```python
from build123d import *

# Parameters (mm, degrees)
SKETCH2_W           = 75
SKETCH2_H           = 50
BOSS_EXTRUDE1_DEPTH = 101.6
CUT_EXTRUDE1_DEPTH  = 101.6
CUT_EXTRUDE2_DEPTH  = 101.6
SKETCH5_W           = 20
SKETCH5_H           = 40
CUT_EXTRUDE3_DEPTH  = 10
SKETCH6_W           = 20
SKETCH6_H           = 40
CUT_EXTRUDE4_DEPTH  = 10
SKETCH7_R           = 2.5
CUT_EXTRUDE5_DEPTH  = 2.5
SKETCH8_R           = 2.5
CUT_EXTRUDE6_DEPTH  = 2.5
CUT_EXTRUDE7_DEPTH  = 121.365392665


with BuildPart() as part:
    # Sketch2 → Boss-Extrude1 (new body)
    with BuildSketch(Plane.XY):
        with Locations((-3.307692308, -6.81353022)):
            Rectangle(SKETCH2_W, SKETCH2_H)
    extrude(amount=BOSS_EXTRUDE1_DEPTH)

    # Sketch3 → Cut-Extrude1 (cut)
    with BuildSketch(Plane(origin=(0, 18.18646978, 0), x_dir=(1, 0, 0), z_dir=(0, 1, 0))):
        Polygon((-40.807692308, -7.5), (-20.807692308, -7.5), (-7.507692308, -20.8), (-7.507692308, -80.8), (-20.807692308, -94.1), (-40.807692308, -94.1), align=None)
    extrude(amount=-CUT_EXTRUDE1_DEPTH, mode=Mode.SUBTRACT)

    # Sketch4 → Cut-Extrude2 (cut)
    with BuildSketch(Plane(origin=(0, 18.18646978, 0), x_dir=(1, 0, 0), z_dir=(0, 1, 0))):
        Polygon((34.192307692, -94.1), (14.192307692, -94.1), (0.892307692, -80.8), (0.892307692, -20.8), (14.192307692, -7.5), (34.192307692, -7.5), align=None)
    extrude(amount=-CUT_EXTRUDE2_DEPTH, mode=Mode.SUBTRACT)

    # Sketch5 → Cut-Extrude3 (cut)
    with BuildSketch(Plane.XY.offset(101.6)):
        with Locations((24.192307692, -6.81353022)):
            Rectangle(SKETCH5_W, SKETCH5_H)
    extrude(amount=-CUT_EXTRUDE3_DEPTH, mode=Mode.SUBTRACT)

    # Sketch6 → Cut-Extrude4 (cut)
    with BuildSketch(Plane.XY.offset(101.6)):
        with Locations((-30.807692308, -6.81353022)):
            Rectangle(SKETCH6_W, SKETCH6_H)
    extrude(amount=-CUT_EXTRUDE4_DEPTH, mode=Mode.SUBTRACT)

    # Sketch7 → Cut-Extrude5 (cut)
    with BuildSketch(Plane.XY.offset(7.5)):
        with Locations((24.192307692, 8.68646978)):
            Circle(SKETCH7_R)
    extrude(amount=-CUT_EXTRUDE5_DEPTH, mode=Mode.SUBTRACT)

    # Sketch8 → Cut-Extrude6 (cut)
    with BuildSketch(Plane.XY.offset(7.5)):
        with Locations((-30.807692308, 8.68646978)):
            Circle(SKETCH8_R)
    extrude(amount=-CUT_EXTRUDE6_DEPTH, mode=Mode.SUBTRACT)

    # Sketch9 → Cut-Extrude7 (cut, through all)
    with BuildSketch(Plane(origin=(0, 18.18646978, 0), x_dir=(1, 0, 0), z_dir=(0, 1, 0))):
        Polygon((-18.24818848, 0), (-3.307692308, -14.940496172), (11.632803865, 0), align=None)
    extrude(amount=-CUT_EXTRUDE7_DEPTH, mode=Mode.SUBTRACT)


solid = part.part
```
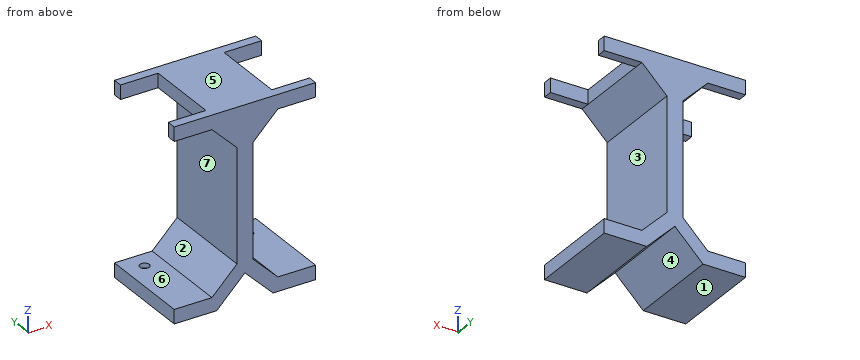
Input: part model. Units: mm. Frame: model coordinates. Face numbers are marked on the shaded views. A direction names the side the tool comes from. Round coordinates to 2 decimals unless told otherwise and drop trailing zeros. Loops run counter-clockwise (first coordinate to the right, second up) from the corner with the lowest first, then second, coordinate; pieces in that order, holes last. Notation, with made-up numbers: (-36, 36.25) -> (16, 36.25) arc R23 cw to (16, 65.25) -> close; hole circle Ø2 at (-21.5, 21). An arc over 180 degrees is marked (long way). Use one line per item in the form item = value. Start each with the question number.
Item 1: Mould query, pull axis Z, two halves, no side actions, for the marked faces 4, 5, 6 and 7. Classes: pulls with the +Z half, pulls with the -Z half, needs draft (parallel to the pull), parting line crosses it, or undercut.
Item 2: Section query C-C on z = 34.5. Return the cut outline in (x, y).
Item 3: Contact query for flat-ended pins moving along their axis: pin 1 Ø4 at (x, y) = (-30.81, 8.69) entering from +Z; pin 2 Ø2 at (y, z) = (-1, 96.5) entering from +X; pin 3 Ø1 at (y, z) = (-11.5, 62) entering from -X. Output: stop coordinate, or through.
Item 4: Material intervals for L1, parallel to Z at x = -24.5, y = -5; L2, parallel to Z at x = -18.5, y = -7; L3, parallel to X at y = 15.5, z = 13.5, sorted ascending. Write a range as from..to.
Item 5: Section query B-B on y = -23.5. Return the cut outline in (x, z).
Item 6: Set-up query: the marked faces 1, 2 and 3. Return all of +Z, -Z, +X, -X, +Y, -Y with unobstructed straight access to the full face (end or side cutting, diameter ignored); none if empty.
Item 7: Section query A-A on x = 19. Return the cut outline in (y, z).
Item 8: Section query D-D on x = -30. Return the cut outline in (y, z), then the cut area to 3 significant figures.
Ans:
q1.face_4 = pulls with the -Z half
q1.face_5 = pulls with the +Z half
q1.face_6 = undercut
q1.face_7 = undercut
q2.outline = (-7.51, -31.81) -> (0.89, -31.81) -> (0.89, 18.19) -> (-7.51, 18.19) -> close
q3.pin_1 = 5
q3.pin_2 = 14.19
q3.pin_3 = -7.51
q4.L1 = 0..7.5
q4.L2 = 0..9.81, 91.79..101.6
q4.L3 = -14.81..-4.75, -1.87..8.19
q5.outline = (-40.81, 0) -> (-18.25, 0) -> (-3.31, 14.94) -> (11.63, 0) -> (34.19, 0) -> (34.19, 7.5) -> (14.19, 7.5) -> (0.89, 20.8) -> (0.89, 80.8) -> (14.19, 94.1) -> (14.19, 101.6) -> (-20.81, 101.6) -> (-20.81, 94.1) -> (-7.51, 80.8) -> (-7.51, 20.8) -> (-20.81, 7.5) -> (-40.81, 7.5) -> close
q6.face_1 = -Z, +X, -X, +Y, -Y
q6.face_2 = -X, +Y, -Y
q6.face_3 = +X, +Y, -Y
q7.outline = (-31.81, 0) -> (18.19, 0) -> (18.19, 7.5) -> (-31.81, 7.5) -> close; (-31.81, 94.1) -> (-26.81, 94.1) -> (-26.81, 101.6) -> (-31.81, 101.6) -> close; (13.19, 94.1) -> (18.19, 94.1) -> (18.19, 101.6) -> (13.19, 101.6) -> close
q8.outline = (-31.81, 0) -> (18.19, 0) -> (18.19, 7.5) -> (11.05, 7.5) -> (11.05, 5) -> (6.32, 5) -> (6.32, 7.5) -> (-31.81, 7.5) -> close; (-31.81, 94.1) -> (-26.81, 94.1) -> (-26.81, 101.6) -> (-31.81, 101.6) -> close; (13.19, 94.1) -> (18.19, 94.1) -> (18.19, 101.6) -> (13.19, 101.6) -> close
q8.area = 438 mm^2
